```python
from build123d import *

# Parameters (mm, degrees)
BOSS_EXTRUDE2_DEPTH = 3.175
SKETCH2_R           = 30
CUT_EXTRUDE1_DEPTH  = 3.175


with BuildPart() as part:
    # Sketch1 → Boss-Extrude2 (new body)
    with BuildSketch(Plane.XY):
        Polygon((-40, 0), (40, 0), (40, 3.175), (76.825, 3.175), (76.825, 25), (80, 25), (80, 75), (76.825, 75), (76.825, 96.825), (40, 96.825), (40, 100), (-40, 100), (-40, 96.825), (-76.825, 96.825), (-76.825, 75), (-80, 75), (-80, 25), (-76.825, 25), (-76.825, 3.175), (-40, 3.175), align=None)
    extrude(amount=BOSS_EXTRUDE2_DEPTH)

    # Sketch2 → Cut-Extrude1 (cut)
    with BuildSketch(Plane.XY.offset(3.175)):
        with Locations((0, 50)):
            Circle(SKETCH2_R)
    extrude(amount=-CUT_EXTRUDE1_DEPTH, mode=Mode.SUBTRACT)


solid = part.part
```
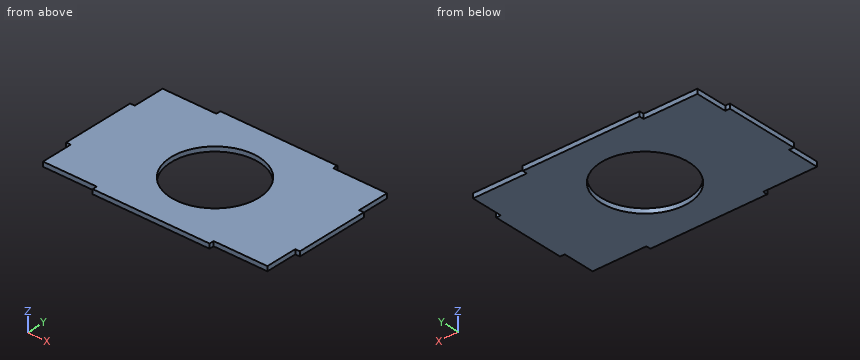
Model file for the job. Use its own axes, mm. Give positions to 0.01 mm unless a question says otherwise; leave off trailing zeros. Order: outer loops, then holes, each group sorted by start corner. A loop starts at its lowest first (then second) coordinate and runs counter-clockwise, first axis right, second up.
1) Saw through at B-B, the plane x = 0. Write the cut outline in (y, z) (3 decimals), then the cut area to 3 significant figures.
2) Saw through at A-A, the plane y = 50. Write the cut outline in (x, z) (3 decimals), then the cut area to 4 significant figures.
3) Saw through at C-C, the plane z = 2.5. Write the cut outline in (x, y) (3 decimals).
4) Saw through at D-D, the plane y = 86. Write the cut outline in (x, z) (3 decimals), then the cut area to 3 significant figures.
5) Pin check, flat tips, straight feed: pin 1 (1.6 mm diameter, centred on x = 79, z = 1.5, fed in from -Y); pin 2 (1 mm diameter, centred on y = 1.5, z = 1, fed in from -X); pin 3 (1.6 mm diameter, centred on x = -58.5, z = 2.5, fed in from +Y) (3 decimals). Stop position of each tip, or through.
6) Wall check: probe 1 along Y at (x, z) = (64, 2.6) (3 decimals); probe 2 along Y at (x, z) = (0, 2.35); probe 3 along X at (y, z) = (18, 2.15) (3 decimals). Give the ranges that are in metal, low to high.
Computed:
1. outline: (0, 0) - (20, 0) - (20, 3.175) - (0, 3.175) - close; (80, 0) - (100, 0) - (100, 3.175) - (80, 3.175) - close
1. area: 127 mm2
2. outline: (-80, 0) - (-30, 0) - (-30, 3.175) - (-80, 3.175) - close; (30, 0) - (80, 0) - (80, 3.175) - (30, 3.175) - close
2. area: 317.5 mm2
3. outline: (-80, 25) - (-76.825, 25) - (-76.825, 3.175) - (-40, 3.175) - (-40, 0) - (40, 0) - (40, 3.175) - (76.825, 3.175) - (76.825, 25) - (80, 25) - (80, 75) - (76.825, 75) - (76.825, 96.825) - (40, 96.825) - (40, 100) - (-40, 100) - (-40, 96.825) - (-76.825, 96.825) - (-76.825, 75) - (-80, 75) - close; hole circle Ø60 at (0, 50)
4. outline: (-76.825, 0) - (76.825, 0) - (76.825, 3.175) - (-76.825, 3.175) - close
4. area: 488 mm2
5. pin 1: stops at y = 25
5. pin 2: stops at x = -40
5. pin 3: stops at y = 96.825
6. probe 1: y = 3.175 to 96.825
6. probe 2: y = 0 to 20, 80 to 100
6. probe 3: x = -76.825 to 76.825
